Check sheet for the modelled part. Datum: model origin and axes. Units: mm. A direction names the side the tool comes from. Give positions to 0.01 mm unless a question says otherwise; leave off trailing zeros. Order: outer loops, then holes, each group sorted by start corner. A loop starts at its lowest first (then second) coordinate and runs counter-clockwise, first axis right, second up.
Item 1: Sectioned sample at B-B on z = 22.5. Record the boundary of the cut face in (x, y), and give its area (3 significant figures).
Item 2: Material ranges on line 1 along Z through (x, y) = (5.7, 8.6) (3 decimals); line 2 along Z through (x, y) = (-12.5, -6.1); line 3 along X through (y, z) = (-6.3, 3), recorded low to high.
Item 3: Sectioned sample at A-A on x = 0. Record the boundary of the cut face in (y, z), and give its area (3 significant figures).
Item 4: Access from +Z, -Z, +X, -X, +Y, -Y to the whole of each face (thin tool, end or side, straight path). Record for faces 1 (the cylindrical face through (-0.054, 8.308, 3.123)), 2 (the flat face through (0, 8, 0.1)), 3 (the cylindrical face through (10.2, 0.1, 14.8)).
Item 5: Sectioned sample at C-C on y = -3. Record the boundary of the cut face in (x, z).
Item 6: Release check for a two-part mould opening along Y. For faces 4 (the flat face through (10.2, -1.8, 6.319)), 5 (the flat face through (3, 8.9, 15)), 6 (the cylindrical face through (-13.79, -6.71, 2.83)) record: released by +Y, released by -Y, zero draft, split by the parting line, or undercut.
Item 7: Gauge pin test, flat ends, axial feed: P1, Ø4, axis at x = -4, z = 23, coming from the -Y side; P2, Ø0.9, axis at x = -10.5, y = -3.5, coming from the -Z side; P3, Ø1.2, axis at y = -7, z = 0.5, coming from the -X side. Record the tip position at first contact, or that the pin passes through.
Item 8: Sectioned sample at D-D on x = 12.5. Record the boundary of the cut face in (y, z), and give its area (3 significant figures).
from build123d import *

# Parameters (mm, degrees)
SALIENTE_EXTRUIR1_DEPTH    = 30
VACIADO1_T                 = 1.2
CROQUIS2_W                 = 41.64599518
CROQUIS2_H                 = 31.401201606
CORTAR_EXTRUIR1_DEPTH      = 1.3
CROQUIS3_W                 = 19.002401527
CROQUIS3_H                 = 2.972205444
CORTAR_EXTRUIR2_DEPTH      = 48.3
CROQUIS4_R                 = 2.75
CROQUIS4_R_2               = 1.3
SALIENTE_EXTRUIR2_DEPTH    = 2
SALIENTE_EXTRUIR2_2_DEPTH  = 2
SALIENTE_EXTRUIR2_3_DEPTH  = 2
SALIENTE_EXTRUIR2_4_DEPTH  = 2
CROQUIS5_W                 = 2.061100057
CROQUIS5_H                 = 29.9
SALIENTE_EXTRUIR3_DEPTH    = 1.5
CROQUIS6_R                 = 1
CORTAR_EXTRUIR3_DEPTH      = 7
CORTAR_EXTRUIR4_DEPTH      = 30
CORTAR_EXTRUIR4_DEPTH_BACK = 32
CROQUIS9_W                 = 7.787362377
CROQUIS9_H                 = 8.000416911


with BuildPart() as part:
    # Croquis1 → Saliente-Extruir1 (new body)
    with BuildSketch(Plane.XY):
        with BuildLine():
            Line((-6.68954408, 7.7), (6.68954408, 7.7))
            ThreePointArc((6.68954408, 7.7), (10.2, 0), (6.68954408, -7.7))
            Line((6.68954408, -7.7), (-6.68954408, -7.7))
            ThreePointArc((-6.68954408, -7.7), (-10.2, 0), (-6.68954408, 7.7))
        make_face()
    extrude(amount=SALIENTE_EXTRUIR1_DEPTH)

    # Vaciado1
    vaciado1_openings = [part.faces().sort_by_distance(p)[0] for p in [
        (0, 0, 30),
    ]]
    offset(amount=VACIADO1_T, openings=vaciado1_openings, kind=Kind.INTERSECTION)

    # Croquis2 → Cortar-Extruir1 (cut)
    with BuildSketch(Plane(origin=(0, 0, -1.2), x_dir=(-1, 0, 0), z_dir=(0, 0, -1))):
        Rectangle(CROQUIS2_W, CROQUIS2_H)
    extrude(amount=-CORTAR_EXTRUIR1_DEPTH, mode=Mode.SUBTRACT)

    # Croquis3 → Cortar-Extruir2 (cut)
    with BuildSketch(Plane.XY.offset(30)):
        with Locations((-0.191367802, -9.186102722)):
            Rectangle(CROQUIS3_W, CROQUIS3_H)
    extrude(amount=-CORTAR_EXTRUIR2_DEPTH, mode=Mode.SUBTRACT)



with BuildPart() as body_2:
    # Croquis4 → Saliente-Extruir2 (new body)
    with BuildSketch(Plane.XZ.offset(7.7)):
        with Locations(Location((12.5, 3, 0), (0, 0, 270))):
            Circle(CROQUIS4_R)
        with Locations(Location((12.5, 3, 0), (0, 0, 270))):
            Circle(CROQUIS4_R_2, mode=Mode.SUBTRACT)
    extrude(amount=-SALIENTE_EXTRUIR2_DEPTH)


with BuildPart() as body_3:
    # Croquis4 → Saliente-Extruir2 2 (new body)
    with BuildSketch(Plane.XZ.offset(7.7)):
        with Locations(Location((12.5, 27, 0), (0, 0, 90))):
            Circle(CROQUIS4_R)
        with Locations(Location((12.5, 27, 0), (0, 0, 90))):
            Circle(CROQUIS4_R_2, mode=Mode.SUBTRACT)
    extrude(amount=-SALIENTE_EXTRUIR2_2_DEPTH)


with BuildPart() as body_4:
    # Croquis4 → Saliente-Extruir2 3 (new body)
    with BuildSketch(Plane.XZ.offset(7.7)):
        with Locations(Location((-12.5, 27, 0), (0, 0, 270))):
            Circle(CROQUIS4_R)
        with Locations(Location((-12.5, 27, 0), (0, 0, 270))):
            Circle(CROQUIS4_R_2, mode=Mode.SUBTRACT)
    extrude(amount=-SALIENTE_EXTRUIR2_3_DEPTH)


with BuildPart() as body_5:
    # Croquis4 → Saliente-Extruir2 4 (new body)
    with BuildSketch(Plane.XZ.offset(7.7)):
        with Locations(Location((-12.5, 3, 0), (0, 0, 90))):
            Circle(CROQUIS4_R)
        with Locations(Location((-12.5, 3, 0), (0, 0, 90))):
            Circle(CROQUIS4_R_2, mode=Mode.SUBTRACT)
    extrude(amount=-SALIENTE_EXTRUIR2_4_DEPTH)


with BuildPart() as part_1:
    add(part.part)

    add(body_2.part)  # Saliente-Extruir3 merges body 2

    add(body_3.part)  # Saliente-Extruir3 merges body 3

    add(body_4.part)  # Saliente-Extruir3 merges body 4

    add(body_5.part)  # Saliente-Extruir3 merges body 5
    # Croquis5 → Saliente-Extruir3 (add)
    with BuildSketch(Plane.XZ.offset(7.7)):
        with Locations((-9.437095098, 15.05)):
            Rectangle(CROQUIS5_W, CROQUIS5_H)
        with Locations((9.437095098, 15.05)):
            Rectangle(CROQUIS5_W, CROQUIS5_H)
    extrude(amount=-SALIENTE_EXTRUIR3_DEPTH)

    # Croquis6 → Cortar-Extruir3 (cut)
    with BuildSketch(Plane(origin=(0, 8.9, 0), x_dir=(1, 0, 0), z_dir=(0, 1, 0))):
        with Locations(Location((5.7, -3.804995741, 0), (0, 0, 180))):
            Circle(CROQUIS6_R)
        with Locations((5.601580803, -26.244572596)):
            Circle(CROQUIS6_R)
        with Locations(Location((-5.7, -3.804995741, 0), (0, 0, 188.292737021))):
            Circle(CROQUIS6_R)
        with Locations(Location((-5.601580803, -26.244572596, 0), (0, 0, 180))):
            Circle(CROQUIS6_R)
        with BuildLine():
            Line((-2.462626263, -24.414792503), (-2.462626263, -5.585207497))
            ThreePointArc((-2.462626263, -5.585207497), (0, -3.122581234), (2.462626263, -5.585207497))
            Line((2.462626263, -5.585207497), (2.462626263, -24.414792503))
            ThreePointArc((2.462626263, -24.414792503), (0, -26.877418766), (-2.462626263, -24.414792503))
        make_face()
        with BuildLine():
            Line((6.616453694, -7.107894038), (6.616453694, -22.942105962))
            ThreePointArc((6.616453694, -22.942105962), (5.7, -23.858559655), (4.783546306, -22.942105962))
            Line((4.783546306, -22.942105962), (4.783546306, -7.107894038))
            ThreePointArc((4.783546306, -7.107894038), (5.7, -6.191440345), (6.616453694, -7.107894038))
        make_face()
        with BuildLine():
            Line((-6.616453694, -7.107894038), (-6.616453694, -22.942105962))
            ThreePointArc((-6.616453694, -22.942105962), (-5.7, -23.858559655), (-4.783546306, -22.942105962))
            Line((-4.783546306, -22.942105962), (-4.783546306, -7.107894038))
            ThreePointArc((-4.783546306, -7.107894038), (-5.7, -6.191440345), (-6.616453694, -7.107894038))
        make_face()
    extrude(amount=-CORTAR_EXTRUIR3_DEPTH, mode=Mode.SUBTRACT)

    # Croquis9 → Cortar-Extruir4 (cut, two sides: drawn at the far end of the back side and taken through both)
    with BuildSketch(Plane(origin=(0, 0, 0), x_dir=(0, 0, -1), z_dir=(1, 0, 0)).offset(-CORTAR_EXTRUIR4_DEPTH_BACK)):
        with Locations((-2.424964561, -1.699791545)):
            Rectangle(CROQUIS9_W, CROQUIS9_H)
        Polygon((-31.528660737, 2.20102722), (-23.741439659, 2.247938616), (-23.693244814, -5.75233313), (-31.480465891, -5.799244526), align=None)
    extrude(amount=CORTAR_EXTRUIR4_DEPTH + CORTAR_EXTRUIR4_DEPTH_BACK, mode=Mode.SUBTRACT)


solid = part_1.part
Report:
1. outline: (-10.47, -7.7) - (-6.69, -7.7) arc R10.2 cw to (-6.69, 7.7) - (-6.62, 7.7) - (-6.62, 8.9) - (-7.12, 8.9) arc R11.4 ccw to (-9.57, -6.2) - (-10.47, -6.2) - close; (-4.78, 7.7) - (-2.46, 7.7) - (-2.46, 8.9) - (-4.78, 8.9) - close; (2.46, 7.7) - (4.78, 7.7) - (4.78, 8.9) - (2.46, 8.9) - close; (6.62, 7.7) - (6.69, 7.7) arc R10.2 cw to (6.69, -7.7) - (10.47, -7.7) - (10.47, -6.2) - (9.57, -6.2) arc R11.4 ccw to (7.12, 8.9) - (6.62, 8.9) - close
1. area: 53.9 mm2
2. line 1: z = 0.1 to 2.805, 4.805 to 6.191, 23.859 to 25.249, 27.24 to 30
2. line 2: z = 0.25 to 1.7, 4.3 to 5.75, 24.25 to 25.7, 28.3 to 29.75
2. line 3: x = -15.25 to -13.8, -11.2 to -8.02, 8.02 to 11.2, 13.8 to 15.25
3. outline: (7.7, 0.1) - (8.9, 0.1) - (8.9, 3.12) - (7.7, 3.12) - close; (7.7, 26.88) - (8.9, 26.88) - (8.9, 30) - (7.7, 30) - close
3. area: 7.37 mm2
4. face 1: +Y, -Y
4. face 2: -Z, +X, -X, +Y, -Y
4. face 3: +Z, -Z
5. outline: (-11, 6.32) - (-9.75, 6.32) - (-9.75, 23.71) - (-11, 23.71) - close; (9.75, 6.32) - (11, 6.32) - (11, 23.71) - (9.75, 23.71) - close
6. face 4: undercut
6. face 5: released by +Y
6. face 6: zero draft
7. P1: stops at y = 7.7
7. P2: stops at z = 6.32
7. P3: stops at x = -14.49
8. outline: (-7.7, 0.25) - (-5.7, 0.25) - (-5.7, 1.7) - (-7.7, 1.7) - close; (-7.7, 4.3) - (-5.7, 4.3) - (-5.7, 5.75) - (-7.7, 5.75) - close; (-7.7, 24.25) - (-5.76, 24.25) - (-5.76, 25.7) - (-7.7, 25.7) - close; (-7.7, 28.3) - (-5.78, 28.3) - (-5.79, 29.75) - (-7.7, 29.75) - close
8. area: 11.4 mm2
